For this review, take the finished solid that the model builds, in its own axes (mm). Coordinates: 2 decimals unless noted, no trailing zeros. Loops run counter-clockwise (first coordinate to the right, second up) from the corner with the lowest first, then second, coordinate; pieces in that order, holes last. Notation, with made-up numbers: M 66.25,-28.5 L 114.25,-28.5 A19 ccw 114.25,7.5 Z; hole C 44.25,5 d3. An arc over 180 degrees is marked long. Answer as a JSON object with one key per item and string values. Group by question number.
Item 1: Add section B-B (z = 14.5). State the section outline as (x, y) points.
Item 2: Wall thickness on L1, parallel to Y at x = 3, z = 10.5; L2, parallel to X at y = 4.75, z = -30; L3, parallel to X at y = 1.5, z = -15: over which ranges is each line inside the solid? List them lowest first. Write a range as from..to.
Item 3: Add section A-A (z = -39). State the section outline as (x, y) points.
Item 4: Insertion check: pin 1 (4 mm diameter, centred on x = 16, z = 27.5, fed in from +Y); pin 2 (1.5 mm diameter, centred on x = 15, y = 6.5, fed in from -Z); pin 3 (1.5 mm diameter, centred on x = 3.5, y = 5.5, fed in from -Z). Each pin has a flat end and moves straight along its axis. Give the tip position at first contact, or say it passes through.
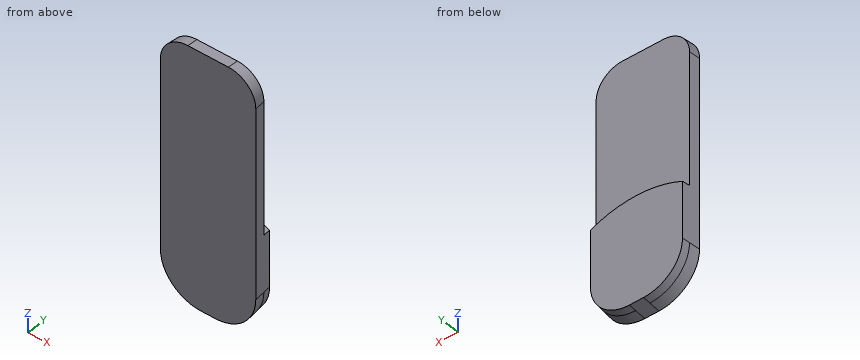
from build123d import *

# Parameters (mm, degrees)
BOSS_EXTRUDE1_DEPTH = 5
BOSS_EXTRUDE1_TAPER = 5
BOSS_EXTRUDE2_DEPTH = 8.5
BOSS_EXTRUDE2_TAPER = 5


with BuildPart() as part:
    # Sketch1 → Boss-Extrude1 (new body)
    with BuildSketch(Plane(origin=(0, 0, 0), x_dir=(1, 0, 0), z_dir=(0, 1, 0))):
        with BuildLine():
            ThreePointArc((-3.25, 59.25), (-16.331475452, 53.831475452), (-21.75, 40.75))
            Line((-21.75, 40.75), (-21.75, -46.75))
            ThreePointArc((-21.75, -46.75), (-18.088834765, -55.588834765), (-9.25, -59.25))
            Line((-9.25, -59.25), (9.25, -59.25))
            ThreePointArc((9.25, -59.25), (18.088834765, -55.588834765), (21.75, -46.75))
            Line((21.75, -46.75), (21.75, 40.75))
            ThreePointArc((21.75, 40.75), (16.331475452, 53.831475452), (3.25, 59.25))
            Line((3.25, 59.25), (-3.25, 59.25))
        make_face()
    extrude(amount=BOSS_EXTRUDE1_DEPTH, taper=BOSS_EXTRUDE1_TAPER)

    # Sketch1<3> → Boss-Extrude2 (add)
    with BuildSketch(Plane(origin=(0, 0, 0), x_dir=(1, 0, 0), z_dir=(0, 1, 0))):
        with BuildLine():
            Line((3.25, 59.25), (-3.25, 59.25))
            ThreePointArc((-3.25, 59.25), (-16.331475452, 53.831475452), (-21.75, 40.75))
            Line((-21.75, 40.75), (-21.75, 14.25))
            ThreePointArc((-21.75, 14.25), (0, 9.271522631), (21.75, 14.25))
            Line((21.75, 14.25), (21.75, 40.75))
            ThreePointArc((21.75, 40.75), (16.331475452, 53.831475452), (3.25, 59.25))
        make_face()
    extrude(amount=BOSS_EXTRUDE2_DEPTH, taper=BOSS_EXTRUDE2_TAPER)


solid = part.part
From the geometry:
{
 "1": {"outline": "M -21.75,0 L 21.75,0 L 21.31,5 L -21.31,5 Z"},
 "2": {"L1": "y = 0..5", "L2": "x = -21.33..21.33", "L3": "x = -21.62..21.62"},
 "3": {"outline": "M -21.75,0 L 21.75,0 L 21.01,8.5 L -21.01,8.5 Z"},
 "4": {"pin 1": "stops at y = 5", "pin 2": "stops at z = -54.92", "pin 3": "stops at z = -58.83"}
}
